Geometry: see drawing. Coordinates: mm, zero at the bounding-box minimum. A direction names the side the tool comes from. Give positions to 0.01 mm unless a question says otherwise; leave off trailing zeros. Loops run counter-clockwise (first coordinate to the right, second up) from the corner with the lowest first, then second, coordinate; pieces in that order, holes last. Notation, with made-up numbers: (24, 54) - (62, 54) arc R21 ccw to (62, 74) - close; hole circle Ø10 at (-21.5, 67.25). An arc over 180 degrees is marked (long way). Use one line per item in the form item = value.
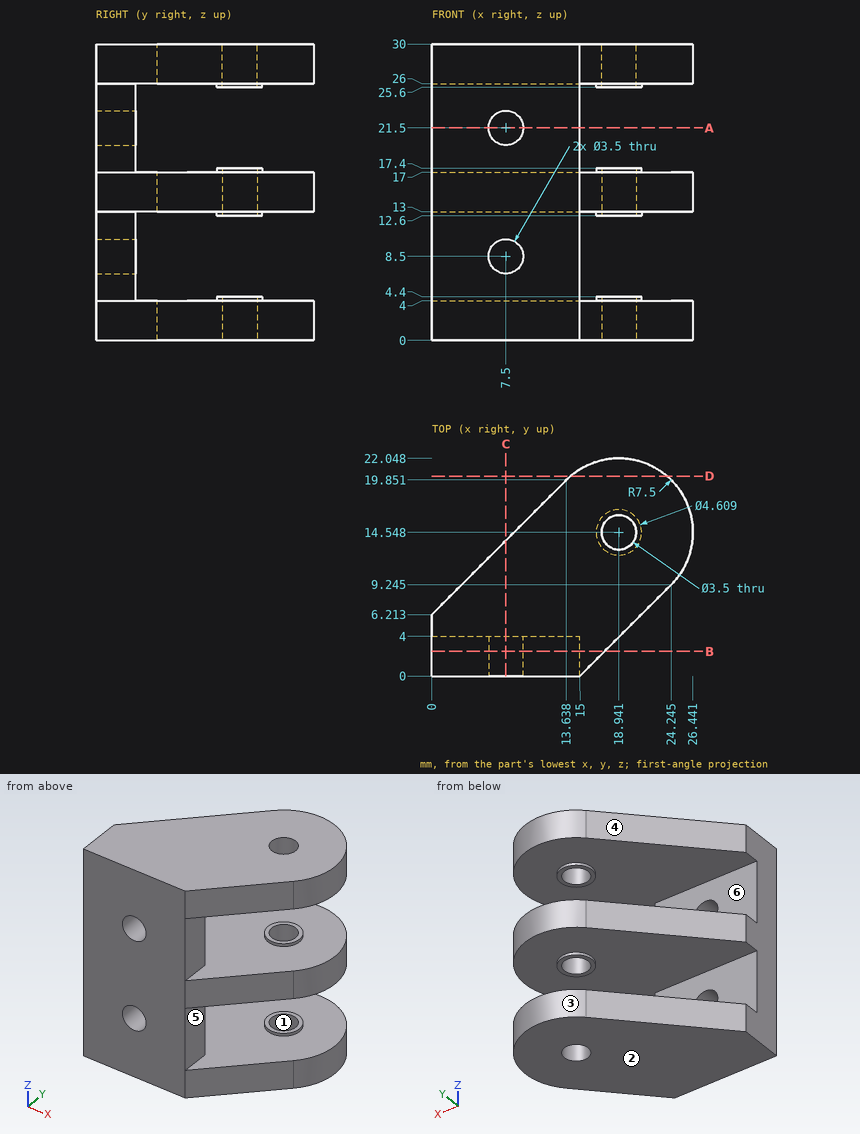
(1) Pin query (flat end, axial travel): P1, Ø3, axis at x = 14.5, z = 14, coming from the +Y side; P2, Ø4, axis at y = 5, z = 12, coming from the +X side; P3, Ø4.5, axis at x = 9, z = 8, coming from the +Y side; P4, Ø6, axis at y = 13, z = 7.5, coming from the +X side. Return the tip coordinate at first contact, or that it passes through.
Solution:
P1 = 21.45
P2 = 21.73
P3 = 4
P4 = through
(2) Access query for the marked faces 4, 5 and 6. Directions: +Z, -Z, +X, -X, +Y, -Y. A direction counts if a zero-diameter tool reaches every point of the face in a straight line with its end or side. Return the directions, or none.
Solution:
face_4 = +Z, -Z, -X, +Y
face_5 = +X, +Y, -Y
face_6 = +X, -X, +Y
(3) Cut plane B-B (y = 2.5). Return the cut outline in (x, z), plus the area to 3 significant figures.
Solution:
outline = (0, 0) - (17.5, 0) - (17.5, 4) - (15, 4) - (15, 13) - (17.5, 13) - (17.5, 17) - (15, 17) - (15, 26) - (17.5, 26) - (17.5, 30) - (0, 30) - close; hole circle Ø3.5 at (7.5, 8.5); hole circle Ø3.5 at (7.5, 21.5)
area = 461 mm2
(4) Material intervals for L1, parallel to Z at x = 24.75, y = 18.5; L2, parallel to Z at x = 7.5, y = 2.1; L3, parallel to Y at x = 13, z = 17.25, sorted ascending. Write a range as from..to.
Solution:
L1 = 0..4, 13..17, 26..30
L2 = 0..6.75, 10.25..19.75, 23.25..30
L3 = 0..4
(5) Cut plane D-D (y = 20.25). Return the cut outline in (x, z), plus the area to 3 significant figures.
Solution:
outline = (14.07, 0) - (23.81, 0) - (23.81, 4) - (14.07, 4) - close; (14.07, 13) - (23.81, 13) - (23.81, 17) - (14.07, 17) - close; (14.07, 26) - (23.81, 26) - (23.81, 30) - (14.07, 30) - close
area = 117 mm2
(6) Pull-direction query (X, two-part tool) for the marked faces 1, 2 and 3; classes: released by +X, released by -X, zero draft, split by the parting line, or undercut.
Solution:
face_1 = undercut
face_2 = zero draft
face_3 = split by the parting line
(7) Cut plane C-C (x = 7.5). Return the cut outline in (y, z).
Solution:
outline = (0, 0) - (13.71, 0) - (13.71, 4) - (4, 4) - (4, 6.75) - (0, 6.75) - close; (0, 10.25) - (4, 10.25) - (4, 13) - (13.71, 13) - (13.71, 17) - (4, 17) - (4, 19.75) - (0, 19.75) - close; (0, 23.25) - (4, 23.25) - (4, 26) - (13.71, 26) - (13.71, 30) - (0, 30) - close
(8) Cut plane A-A (z = 21.5). Return the cut outline in (x, y).
Solution:
outline = (0, 0) - (5.75, 0) - (5.75, 4) - (0, 4) - close; (9.25, 0) - (15, 0) - (15, 4) - (9.25, 4) - close
